Can you work these out from the drawing? Everything is in mm from the part's minimum corner. Give positions to 0.01 mm unless a question says otherwise; leave off trailing zeros. Order: outer loops, then holes, each group sorted by start corner. A loop starts at its lowest first (then second) coordinate and runs counter-clockwise, first axis right, second up. Notation, with made-up numbers: (-31, 83) - (-1, 83) arc R15 ccw to (-1, 99) - close; hole circle Ø7 at (87, 46). An arc over 180 degrees is marked (long way). One line per question, with ' | ' between items.
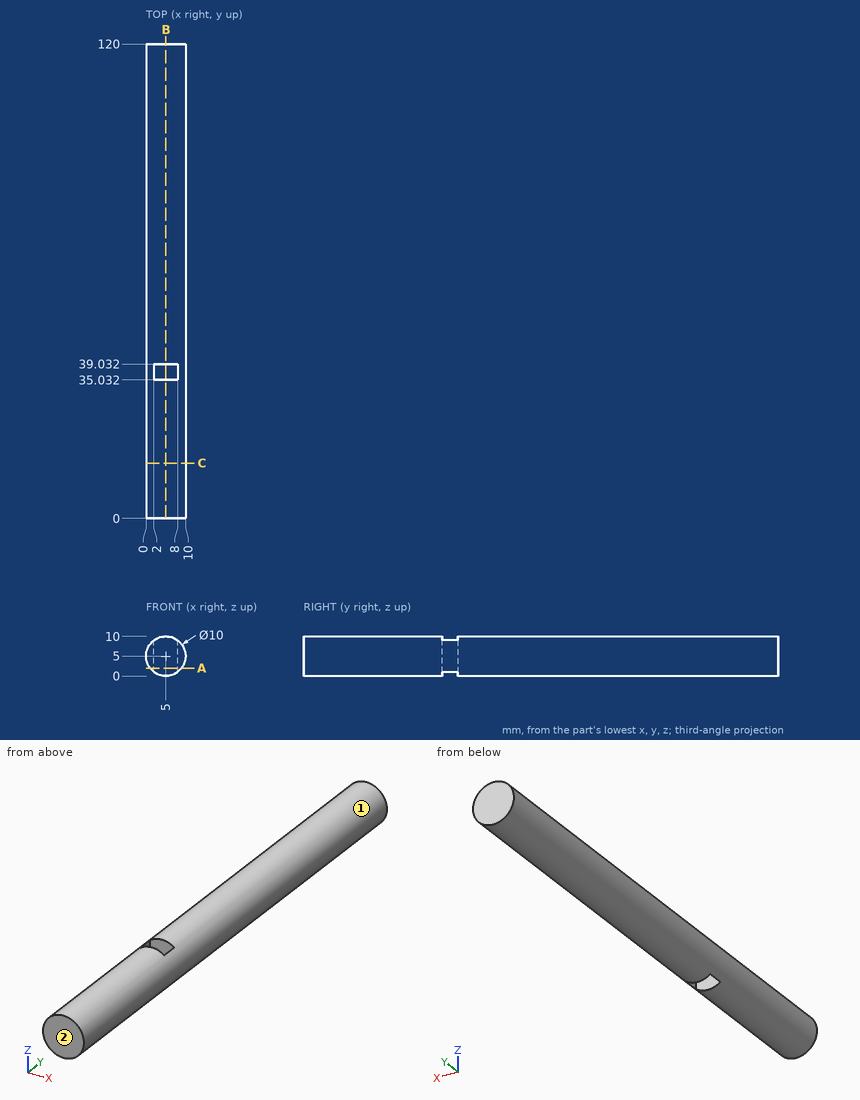
(1) Imagine slicing it at C-C (y = 14). List the corners of the cut face in (x, z) for me.
Answer below:
outline: circle Ø10 at (5, 5)
(2) Will these pins go through, and if not, where does the flat tip stop? pin 1 (1 mm diameter, centred on y = 13.5, z = 2, fed in from -X); pin 2 (1 mm diameter, centred on x = 1.5, y = 51.5, fed in from +Z); pin 3 (4 mm diameter, centred on x = 1.5, y = 63, fed in from +Z).
Answer below:
pin 1: x = 0.67 | pin 2: z = 9 | pin 3: z = 9.77
(3) Imagine slicing it at A-A (z = 2). List the corners of the cut face in (x, y) for me.
Answer below:
outline: (1, 0) - (9, 0) - (9, 120) - (1, 120) - close; hole (2, 35.03) - (8, 35.03) - (8, 39.03) - (2, 39.03) - close
(4) If I drill on line 1 (Y direction, x = 4.75, z = 1.5); line 2 (X direction, y = 66, z = 4.75); line 3 (X direction, y = 11.5, z = 1), over which ranges is the centre line in solid material (lowest first)?
Answer below:
line 1: 0 to 35.03, 39.03 to 120 | line 2: 0.01 to 9.99 | line 3: 2 to 8
(5) Imagine slicing it at B-B (x = 5). List the corners of the cut face in (y, z) for me, and give its area (3 significant figures).
Answer below:
outline: (0, 0) - (35.03, 0) - (35.03, 10) - (0, 10) - close; (39.03, 0) - (120, 0) - (120, 10) - (39.03, 10) - close | area: 1,160 mm^2
(6) If we mould it in two halves opening along X, with no side actions, what happens to the marked faces 1 and 2? For each: released by +X, released by -X, zero draft, split by the parting line, or undercut.
Answer below:
face 1: split by the parting line | face 2: zero draft
